Input: part model. Units: mm. Frame: model coordinates. A direction names the side the tool comes from. Coordinates: 2 decimals unless noted, no trailing zeros. Order: outer loops, then holes, each group sorted by start corner. A loop starts at its lowest first (then second) coordinate and runs counter-clockwise, first axis right, second up. Notation, with made-up numbers: (58, 68) - (80, 68) arc R3 cw to (80, 73) - close; hole circle Ø11 at (-16.5, -17). An arc over 180 degrees is marked (long way). Answer as CSV lines item,"result". Start each with the question number.
Item 1: Draft query along Z for faces 1 (the cylindrical face through (-35.4, 1.97, -13.43)), 2 (the flat face through (-45, 2, 14)), 3 (the cylindrical face through (-47.372, 1.972, 3.467)). Return one class per face: +Z half, -Z half, draft (parallel to the pull), parting line (faces both ways), or undercut.
Item 2: Material intervals for line 1 along X through (y, z) = (2.8, 0); line 2 along X through (y, z) = (3.15, -7.5); line 3 along X through (y, z) = (0.5, 4.25), sorted ascending.
Item 3: Section A-A (x = -50.8). Output: boundary loops of the cut face in (y, z).
Item 4: Section C-C (y = 1.9). State how many separate pieces and enclosed holes the cut face has, and give its area (3 significant figures).
Item 5: Section B-B (z = 0). Output: boundary loops of the cut face in (x, y).
Item 6: First-contact query: pin 1 (1.5 mm diameter, centred on x = 42.5, y = 1, fed in from -Z); pin 2 (6 mm diameter, centred on x = -50.8, z = 0, fed in from -Y); pin 3 (1 mm diameter, centred on y = 1.5, z = -5.5, fed in from -X). Flat tips, straight axial feed; report the tip coordinate or a pass-through.
Item 7: Section D-D (x = 38.1). Output: boundary loops of the cut face in (y, z).
Item 8: Access query for faces 4 (the flat face through (10, 2, 5.915)), 5 (the flat face through (-44.1, 1.97, 4.93)), 6 (the cylindrical face through (-34.23, 1.972, -6.516)). Directions: +Z, -Z, +X, -X, +Y, -Y. A direction counts if a zero-diameter tool reaches every point of the face in a straight line with its end or side. Return the directions, or none.
from build123d import *

# Parameters (mm, degrees)
SKETCH1_R           = 3.25
SKETCH1_R_2         = 2.38125
BOSS_EXTRUDE1_DEPTH = 4
SKETCH2_R           = 1.5875
CUT_EXTRUDE1_DEPTH  = 10


with BuildPart() as part:
    # Sketch1 → Boss-Extrude1 (new body)
    with BuildSketch(Plane(origin=(0, 0, 0), x_dir=(1, 0, 0), z_dir=(0, 1, 0))):
        with BuildLine():
            Line((-50.8, 14), (-36.8, 14))
            ThreePointArc((-36.8, 14), (-35.385786438, 13.414213562), (-34.8, 12))
            Line((-34.8, 12), (-34.8, 7.914556152))
            ThreePointArc((-34.8, 7.914556152), (-34.214213562, 6.500342589), (-32.8, 5.914556152))
            Line((-32.8, 5.914556152), (50.8, 5.914556152))
            ThreePointArc((50.8, 5.914556152), (56.714556152, 0), (50.8, -5.914556152))
            Line((50.8, -5.914556152), (-32.8, -5.914556152))
            ThreePointArc((-32.8, -5.914556152), (-34.214213562, -6.500342589), (-34.8, -7.914556152))
            Line((-34.8, -7.914556152), (-34.8, -12))
            ThreePointArc((-34.8, -12), (-35.385786438, -13.414213562), (-36.8, -14))
            Line((-36.8, -14), (-50.8, -14))
            Line((-50.8, -14), (-52.8, -14))
            ThreePointArc((-52.8, -14), (-66.8, 0), (-52.8, 14))
            Line((-52.8, 14), (-50.8, 14))
        make_face()
        with Locations(Location((-50.8, 0, 0), (0, 0, 270))):
            Circle(SKETCH1_R, mode=Mode.SUBTRACT)
        with Locations(Location((50.8, 0, 0), (0, 0, 270))):
            Circle(SKETCH1_R_2, mode=Mode.SUBTRACT)
        with BuildLine():
            Line((-57.252349378, 8.220116331), (-54.247145558, 5.214912511))
            ThreePointArc((-54.247145558, 5.214912511), (-54.247145558, 3.447145558), (-56.014912511, 3.447145558))
            Line((-56.014912511, 3.447145558), (-59.020116331, 6.452349378))
            ThreePointArc((-59.020116331, 6.452349378), (-59.020116331, 8.220116331), (-57.252349378, 8.220116331))
        make_face(mode=Mode.SUBTRACT)
        with BuildLine():
            Line((-42.579883669, 6.452349378), (-45.585087489, 3.447145558))
            ThreePointArc((-45.585087489, 3.447145558), (-47.352854442, 3.447145558), (-47.352854442, 5.214912511))
            Line((-47.352854442, 5.214912511), (-44.347650622, 8.220116331))
            ThreePointArc((-44.347650622, 8.220116331), (-42.579883669, 8.220116331), (-42.579883669, 6.452349378))
        make_face(mode=Mode.SUBTRACT)
        with BuildLine():
            Line((-44.347650622, -8.220116331), (-47.352854442, -5.214912511))
            ThreePointArc((-47.352854442, -5.214912511), (-47.352854442, -3.447145558), (-45.585087489, -3.447145558))
            Line((-45.585087489, -3.447145558), (-42.579883669, -6.452349378))
            ThreePointArc((-42.579883669, -6.452349378), (-42.579883669, -8.220116331), (-44.347650622, -8.220116331))
        make_face(mode=Mode.SUBTRACT)
        with BuildLine():
            Line((-59.020116331, -6.452349378), (-56.014912511, -3.447145558))
            ThreePointArc((-56.014912511, -3.447145558), (-54.247145558, -3.447145558), (-54.247145558, -5.214912511))
            Line((-54.247145558, -5.214912511), (-57.252349378, -8.220116331))
            ThreePointArc((-57.252349378, -8.220116331), (-59.020116331, -8.220116331), (-59.020116331, -6.452349378))
        make_face(mode=Mode.SUBTRACT)
    extrude(amount=BOSS_EXTRUDE1_DEPTH)

    # Sketch2 → Cut-Extrude1 (cut)
    with BuildSketch(Plane.XZ):
        with Locations(Location((38.1, 0, 0), (0, 0, 270))):
            Circle(SKETCH2_R)
    extrude(amount=-CUT_EXTRUDE1_DEPTH, mode=Mode.SUBTRACT)


solid = part.part
Determined:
1,face 1,"-Z half"
1,face 2,"+Z half"
1,face 3,"undercut"
2,line 1,"x = -66.8 to -54.05, -47.55 to 36.51, 39.69 to 48.42, 53.18 to 56.71"
2,line 2,"x = -64.62 to -59.38, -56.53 to -45.07, -42.22 to -34.76"
2,line 3,"x = -66.14 to -56.82, -53.88 to -47.72, -44.78 to 54.91"
3,outline,"(0, -14) - (4, -14) - (4, -3.25) - (0, -3.25) - close; (0, 3.25) - (4, 3.25) - (4, 14) - (0, 14) - close"
4,separate pieces,"1"
4,enclosed holes,"7"
4,area,"1,760 mm^2"
5,outline,"(-66.8, 0) - (-54.05, 0) - (-54.05, 4) - (-66.8, 4) - close; (-47.55, 0) - (36.51, 0) - (36.51, 4) - (-47.55, 4) - close; (39.69, 0) - (48.42, 0) - (48.42, 4) - (39.69, 4) - close; (53.18, 0) - (56.71, 0) - (56.71, 4) - (53.18, 4) - close"
6,pin 1,"stops at z = -5.91"
6,pin 2,"passes through"
6,pin 3,"stops at x = -65.88"
7,outline,"(0, -5.91) - (4, -5.91) - (4, -1.59) - (0, -1.59) - close; (0, 1.59) - (4, 1.59) - (4, 5.91) - (0, 5.91) - close"
8,face 4,"+Z, +X, +Y, -Y"
8,face 5,"+Y, -Y"
8,face 6,"-Z, +X, +Y, -Y"
